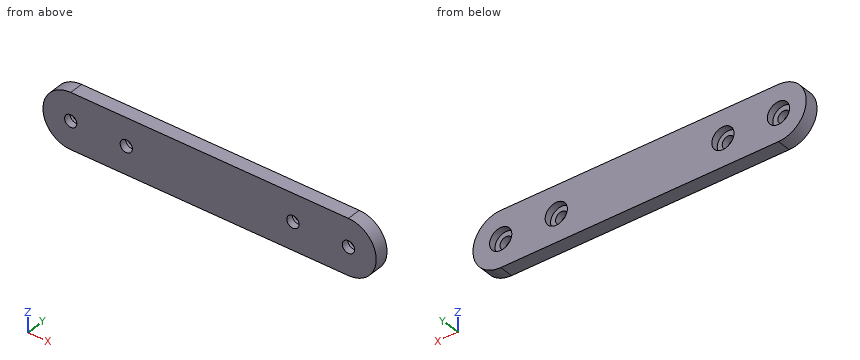
```python
from build123d import *

# Parameters (mm, degrees)
SKETCH1_R           = 2.794
SKETCH1_R_2         = 2.813515076
BOSS_EXTRUDE1_DEPTH = 6.35
SKETCH3_R           = 2.794
CUT_EXTRUDE2_DEPTH  = 6.35
SKETCH2_R           = 5.08
CUT_EXTRUDE1_DEPTH  = 3.175


with BuildPart() as part:
    # Sketch1 → Boss-Extrude1 (new body)
    with BuildSketch(Plane(origin=(0, 0, 0), x_dir=(1, 0, 0), z_dir=(0, 1, 0))):
        with BuildLine():
            Line((0, 12.7), (127, 12.7))
            ThreePointArc((127, 12.7), (139.7, 0), (127, -12.7))
            Line((127, -12.7), (0, -12.7))
            ThreePointArc((0, -12.7), (-12.7, 0), (0, 12.7))
        make_face()
        with Locations(Location((0, 0, 0), (0, 0, 270))):
            Circle(SKETCH1_R, mode=Mode.SUBTRACT)
        with Locations(Location((127, 0, 0), (0, 0, 270))):
            Circle(SKETCH1_R_2, mode=Mode.SUBTRACT)
    extrude(amount=BOSS_EXTRUDE1_DEPTH)

    # Sketch3 → Cut-Extrude2 (cut)
    with BuildSketch(Plane(origin=(0, 6.35, 0), x_dir=(1, 0, 0), z_dir=(0, 1, 0))):
        with Locations(Location((25.4, 0, 0), (0, 0, 270))):
            Circle(SKETCH3_R)
        with Locations(Location((101.6, 0, 0), (0, 0, 270))):
            Circle(SKETCH3_R)
    extrude(amount=-CUT_EXTRUDE2_DEPTH, mode=Mode.SUBTRACT)

    # Sketch2 → Cut-Extrude1 (cut)
    with BuildSketch(Plane(origin=(0, 6.35, 0), x_dir=(1, 0, 0), z_dir=(0, 1, 0))):
        with Locations(Location((0, 0, 0), (0, 0, 270))):
            Circle(SKETCH2_R)
        with Locations(Location((127, 0, 0), (0, 0, 270))):
            Circle(SKETCH2_R)
        with Locations(Location((25.4, 0, 0), (0, 0, 270))):
            Circle(SKETCH2_R)
        with Locations(Location((101.6, 0, 0), (0, 0, 270))):
            Circle(SKETCH2_R)
    extrude(amount=-CUT_EXTRUDE1_DEPTH, mode=Mode.SUBTRACT)


solid = part.part
```
Check sheet for the modelled part. Datum: model origin and axes. Units: mm. Coordinates: 2 decimals unless noted, no trailing zeros. Loops run counter-clockwise (first coordinate to the right, second up) from the corner with the lowest first, then second, coordinate; pieces in that order, holes last. Notation, with made-up numbers: M -12.5,4 L 26.5,4 A19 cw 26.5,30 Z; hole C 37.25,85.25 d9. An arc over 180 degrees is marked long. Answer as a JSON object with one key per item and string values.
1. Depth check by flat-ended pin: P1, Ø5, axis at x = 125.5, z = -2.5, coming from the +Y side; P2, Ø4.5, axis at x = 0, z = 0, coming from the -Y side; P3, Ø6.5, axis at x = 25.4, z = 0, coming from the +Y side (3 decimals). Enter the tip coordinate at first touch or a pass-through.
Outcome:
{"P1": "y = 6.35", "P2": "through", "P3": "y = 3.175"}
2. Sectioned sample at B-B on y = 4.25. Record the cut outline in (x, z).
Outcome:
{"outline": "M 0,-12.7 L 127,-12.7 A12.7 ccw 127,12.7 L 0,12.7 A12.7 ccw Z; hole C 0,0 d10.16; hole C 25.4,0 d10.16; hole C 101.6,0 d10.16; hole C 127,0 d10.16"}
3. Sectioned sample at A-A on x = 101.6. Record the cut outline in (y, z) (3 decimals).
Outcome:
{"outline": "M 0,-12.7 L 6.35,-12.7 L 6.35,-5.08 L 3.175,-5.08 L 3.175,-2.794 L 0,-2.794 Z; M 0,2.794 L 3.175,2.794 L 3.175,5.08 L 6.35,5.08 L 6.35,12.7 L 0,12.7 Z"}
4. Scan lines: L1, parallel to X at y = 1.2, z = 0; L2, parallel to X at y = 3.9, z = 0; L3, parallel to Z at x = 131, y = 6. Record each from-to range of solid material in increasing order. Write a range as from..to.
Outcome:
{"L1": "-12.7..-2.79, 2.79..22.61, 28.19..98.81, 104.39..124.19, 129.81..139.7", "L2": "-12.7..-5.08, 5.08..20.32, 30.48..96.52, 106.68..121.92, 132.08..139.7", "L3": "-12.05..-3.13, 3.13..12.05"}
5. Sectioned sample at C-C on z = 0. Count the separate pieces of the cut face and the enclosed holes in it, and give its area (3 significant figures).
Outcome:
{"separate pieces": "5", "enclosed holes": "0", "area": "768 mm²"}
6. Sectioned sample at D-D on z = 10.75. Record the cut outline in (x, y).
Outcome:
{"outline": "M -6.76,0 L 133.76,0 L 133.76,6.35 L -6.76,6.35 Z"}
